Source: CAD feature listing. Evaluate the final solid. Frame: model axes, mm. Face numbers are marked on the shaded views. A direction names the side the tool comes from. Round coordinates to 2 decimals unless told otherwise and drop trailing zeros. Write each loop counter-clockwise with the first axis right and the second up, starting at its lowest first coordinate (ties: lowest second). Pieces come first, ordered by that corner, then holes.
```python
from build123d import *

# Parameters (mm, degrees)
SKETCH1_W           = 50
SKETCH1_H           = 170
BOSS_EXTRUDE1_DEPTH = 55
SKETCH2_W           = 34
SKETCH2_H           = 27
CUT_EXTRUDE1_DEPTH  = 181.416185527
SKETCH3_W           = 10
SKETCH3_H           = 24
SKETCH3_R           = 4.25
SKETCH3_R_2         = 1
CUT_EXTRUDE2_DEPTH  = 186.539753153
SKETCH4_W           = 2
SKETCH4_H           = 24
CUT_EXTRUDE3_DEPTH  = 178.623196683
SKETCH5_W           = 6.25
SKETCH5_H           = 11.25
CUT_EXTRUDE4_DEPTH  = 186.539753153
SKETCH6_W           = 38
SKETCH6_H           = 10
CUT_EXTRUDE5_DEPTH  = 181.416185527
SKETCH8_W           = 13.25
SKETCH8_H           = 2.25
CUT_EXTRUDE7_DEPTH  = 186.539753153
SKETCH9_W           = 34
SKETCH9_H           = 35.25
CUT_EXTRUDE8_DEPTH  = 179.297679458
SKETCH11_W          = 13.25
SKETCH11_H          = 20.25
CUT_EXTRUDE9_DEPTH  = 184.480414486
SKETCH12_W          = 28.5
SKETCH12_H          = 15
BOSS_EXTRUDE2_DEPTH = 8
SKETCH14_W          = 34
SKETCH14_H          = 15
SKETCH14_H_2        = 10.25
BOSS_EXTRUDE3_DEPTH = 13.25
SKETCH16_R          = 4.5
SKETCH16_R_2        = 2.5
CUT_EXTRUDE13_DEPTH = 8


with BuildPart() as part:
    # Sketch1 → Boss-Extrude1 (new body)
    with BuildSketch(Plane.XY):
        with Locations((0, -85)):
            Rectangle(SKETCH1_W, SKETCH1_H)
    extrude(amount=-BOSS_EXTRUDE1_DEPTH)

    # Sketch2 → Cut-Extrude1 (cut, through all)
    with BuildSketch(Plane.XY):
        with Locations((0, -13.5)):
            Rectangle(SKETCH2_W, SKETCH2_H)
    extrude(amount=-CUT_EXTRUDE1_DEPTH, mode=Mode.SUBTRACT)

    # Sketch3 → Cut-Extrude2 (cut, through all)
    with BuildSketch(Plane(origin=(25, 0, 0), x_dir=(0, 0, -1), z_dir=(1, 0, 0))):
        with Locations((50, -12)):
            Rectangle(SKETCH3_W, SKETCH3_H)
        with Locations((5, -12)):
            Rectangle(SKETCH3_W, SKETCH3_H)
        with Locations(Location((27.5, -12.75, 0), (0, 0, 90))):
            Circle(SKETCH3_R)
        with Locations(Location((35.5, -12.75, 0), (0, 0, 90))):
            Circle(SKETCH3_R_2)
        with Locations(Location((27.5, -4.75, 0), (0, 0, 90))):
            Circle(SKETCH3_R_2)
        with Locations(Location((27.5, -20.75, 0), (0, 0, 90))):
            Circle(SKETCH3_R_2)
        with Locations(Location((19.5, -12.75, 0), (0, 0, 90))):
            Circle(SKETCH3_R_2)
    extrude(amount=-CUT_EXTRUDE2_DEPTH, mode=Mode.SUBTRACT)

    # Sketch4 → Cut-Extrude3 (cut, through all)
    with BuildSketch(Plane.XY.offset(-10)):
        with Locations((-18, -12)):
            Rectangle(SKETCH4_W, SKETCH4_H)
        with Locations((18, -12)):
            Rectangle(SKETCH4_W, SKETCH4_H)
    extrude(amount=-CUT_EXTRUDE3_DEPTH, mode=Mode.SUBTRACT)

    # Sketch5 → Cut-Extrude4 (cut, through all)
    with BuildSketch(Plane(origin=(25, 0, 0), x_dir=(0, 0, -1), z_dir=(1, 0, 0))):
        with BuildLine():
            Line((45, 0), (10, 0))
            Line((10, 0), (10, -12.75))
            Line((10, -12.75), (16.25, -12.75))
            ThreePointArc((16.25, -12.75), (27.5, -1.5), (38.75, -12.75))
            Line((38.75, -12.75), (45, -12.75))
            Line((45, -12.75), (45, 0))
        make_face()
        with Locations((13.125, -18.375)):
            Rectangle(SKETCH5_W, SKETCH5_H)
        with Locations((41.875, -18.375)):
            Rectangle(SKETCH5_W, SKETCH5_H)
    extrude(amount=-CUT_EXTRUDE4_DEPTH, mode=Mode.SUBTRACT)

    # Sketch6 → Cut-Extrude5 (cut, through all)
    with BuildSketch(Plane.XY):
        with Locations((0, -29)):
            Rectangle(SKETCH6_W, SKETCH6_H)
    extrude(amount=-CUT_EXTRUDE5_DEPTH, mode=Mode.SUBTRACT)

    # Sketch8 → Cut-Extrude7 (cut, through all)
    with BuildSketch(Plane(origin=(25, 0, 0), x_dir=(0, 0, -1), z_dir=(1, 0, 0))):
        with BuildLine():
            Line((27.5, -157.5), (27.5, -132.5))
            Line((27.5, -132.5), (13.25, -132.5))
            Line((13.25, -132.5), (13.25, -167.75))
            Line((13.25, -167.75), (17.25, -167.75))
            ThreePointArc((17.25, -167.75), (20.252155493, -160.502155493), (27.5, -157.5))
        make_face()
        with BuildLine():
            Line((41.75, -167.75), (41.75, -132.5))
            Line((41.75, -132.5), (27.5, -132.5))
            Line((27.5, -132.5), (27.5, -157.5))
            ThreePointArc((27.5, -157.5), (34.747844507, -160.502155493), (37.75, -167.75))
            Line((37.75, -167.75), (41.75, -167.75))
        make_face()
        with Locations((48.375, -168.875)):
            Rectangle(SKETCH8_W, SKETCH8_H)
        with Locations((6.625, -168.875)):
            Rectangle(SKETCH8_W, SKETCH8_H)
        with BuildLine():
            Line((17.25, -167.75), (13.25, -167.75))
            Line((13.25, -167.75), (13.25, -170))
            Line((13.25, -170), (17.5, -170))
            ThreePointArc((17.5, -170), (17.31269172, -168.881923142), (17.25, -167.75))
        make_face()
        with BuildLine():
            Line((41.75, -170), (41.75, -167.75))
            Line((41.75, -167.75), (37.75, -167.75))
            ThreePointArc((37.75, -167.75), (37.68730828, -168.881923142), (37.5, -170))
            Line((37.5, -170), (41.75, -170))
        make_face()
        with BuildLine():
            Line((27.5, -167.75), (27.5, -157.5))
            ThreePointArc((27.5, -157.5), (20.252155493, -160.502155493), (17.25, -167.75))
            Line((17.25, -167.75), (27.5, -167.75))
        make_face()
        with BuildLine():
            ThreePointArc((37.75, -167.75), (34.747844507, -160.502155493), (27.5, -157.5))
            Line((27.5, -157.5), (27.5, -167.75))
            Line((27.5, -167.75), (37.75, -167.75))
        make_face()
        with BuildLine():
            Line((27.5, -170), (27.5, -167.75))
            Line((27.5, -167.75), (17.25, -167.75))
            ThreePointArc((17.25, -167.75), (17.31269172, -168.881923142), (17.5, -170))
            Line((17.5, -170), (27.5, -170))
        make_face()
        with BuildLine():
            ThreePointArc((37.5, -170), (37.68730828, -168.881923142), (37.75, -167.75))
            Line((37.75, -167.75), (27.5, -167.75))
            Line((27.5, -167.75), (27.5, -170))
            Line((27.5, -170), (37.5, -170))
        make_face()
    extrude(amount=-CUT_EXTRUDE7_DEPTH, mode=Mode.SUBTRACT)

    # Sketch9 → Cut-Extrude8 (cut, through all)
    with BuildSketch(Plane.XY):
        with Locations((0, -150.125)):
            Rectangle(SKETCH9_W, SKETCH9_H)
    extrude(amount=-CUT_EXTRUDE8_DEPTH, mode=Mode.SUBTRACT)

    # Sketch11 → Cut-Extrude9 (cut, through all)
    with BuildSketch(Plane(origin=(25, 0, 0), x_dir=(0, 0, -1), z_dir=(1, 0, 0))):
        with BuildLine():
            ThreePointArc((17.25, -167.75), (20.252155493, -160.502155493), (27.5, -157.5))
            Line((27.5, -157.5), (27.5, -147.5))
            Line((27.5, -147.5), (13.25, -147.5))
            Line((13.25, -147.5), (13.25, -167.75))
            Line((13.25, -167.75), (17.25, -167.75))
        make_face()
        with BuildLine():
            Line((27.5, -147.5), (27.5, -157.5))
            ThreePointArc((27.5, -157.5), (34.747844507, -160.502155493), (37.75, -167.75))
            Line((37.75, -167.75), (41.75, -167.75))
            Line((41.75, -167.75), (41.75, -147.5))
            Line((41.75, -147.5), (27.5, -147.5))
        make_face()
        with Locations((48.375, -157.625)):
            Rectangle(SKETCH11_W, SKETCH11_H)
        with Locations((6.625, -157.625)):
            Rectangle(SKETCH11_W, SKETCH11_H)
    extrude(amount=-CUT_EXTRUDE9_DEPTH, mode=Mode.SUBTRACT)

    # Sketch12 → Boss-Extrude2 (add)
    with BuildSketch(Plane(origin=(25, 0, 0), x_dir=(0, 0, -1), z_dir=(1, 0, 0))):
        with Locations((27.5, -140)):
            Rectangle(SKETCH12_W, SKETCH12_H)
    boss_extrude2 = extrude(amount=-BOSS_EXTRUDE2_DEPTH)

    # Mirror1: Boss-Extrude2 across plane
    add(boss_extrude2.mirror(Plane(origin=(0, 0, 0), x_dir=(0, 0, 1), z_dir=(1, 0, 0))))

    # Sketch14 → Boss-Extrude3 (add)
    with BuildSketch(Plane.XY):
        with Locations((0, -140)):
            Rectangle(SKETCH14_W, SKETCH14_H)
        with Locations((0, -152.625)):
            Rectangle(SKETCH14_W, SKETCH14_H_2)
    boss_extrude3 = extrude(amount=-BOSS_EXTRUDE3_DEPTH)

    # Mirror2: Boss-Extrude3 across plane
    add(boss_extrude3.mirror(Plane.XY.offset(-27.5)))

    # Sketch16 → Cut-Extrude13 (cut)
    # profile 1 of 3: a face of its own
    with BuildSketch(Plane(origin=(25, 0, 0), x_dir=(0, 0, -1), z_dir=(1, 0, 0))):
        with Locations(Location((16.5, -135.75, 0), (0, 0, 90))):
            Circle(SKETCH16_R)
        with Locations((16.5, -135.75)):
            Circle(SKETCH16_R_2, mode=Mode.SUBTRACT)
    # profile 2 of 3: a face of its own
    with BuildSketch(Plane(origin=(25, 0, 0), x_dir=(0, 0, -1), z_dir=(1, 0, 0))):
        with Locations((16.5, -135.75)):
            Circle(SKETCH16_R_2)
    # profile 3 of 3: a face of its own
    with BuildSketch(Plane(origin=(25, 0, 0), x_dir=(0, 0, -1), z_dir=(1, 0, 0))):
        with Locations(Location((38.5, -135.75, 0), (0, 0, 90))):
            Circle(SKETCH16_R)
    cut_extrude13 = extrude(amount=-CUT_EXTRUDE13_DEPTH, mode=Mode.SUBTRACT)

    # Mirror3: Cut-Extrude13 across plane
    add(cut_extrude13.mirror(Plane(origin=(0, 0, 0), x_dir=(0, 0, 1), z_dir=(1, 0, 0))), mode=Mode.SUBTRACT)


solid = part.part
```
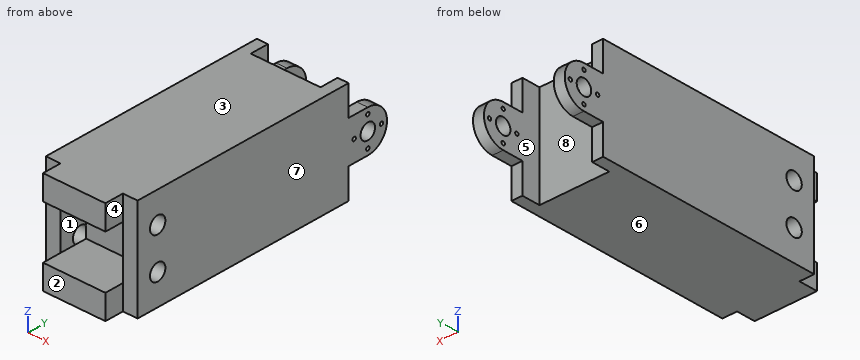
Q1. Set-up query: the marked faces 1, 2, 3, 4 and 5. Return all of +Z, -Z, +X, -X, +Y, -Y with unobstructed straight access to the full face (end or side cutting, diameter ignored); none if empty.
Q2. Pin query (flat end, axial travel): P1, Ø5, axis at x = -22.5, y = -20.5, coming from the -Z side; P2, Ø4, axis at x = -7.5, z = -44, coming from the +Y side; P3, Ø8, axis at y = -152.5, z = -50, coming from the -X side; P4, Ø1.4, axis at y = -135.5, z = -12.5, coming from the +X side. Return the tip coordinate at first contact, or that it passes through.
Q3. Section query C-C, the plane y = -144.5. Output: boundary loops of the cut face in (x, z).
Q4. Section query A-A, the plane z = -7.5. Output: boundary loops of the cut face in (x, y).
Q5. Line query: line 1 (Z direction, x = -20, y = -135); line 2 (Z direction, x = 10.5, y = -142); line 3 (Y direction, x = 21, z = -35). Output: solid intervals per line, ascending.
Q6. Section query B-B, the plane x = 10.5. Output: boundary loops of the cut face in (y, z), and give its area (3 significant figures).
Q7. Mould query, pull axis X, two halves, no side actions, for the marked faces 6, 7 and 8. Classes: pulls with the +X half, pulls with the -X half, needs draft (parallel to the pull), parting line crosses it, or undercut.
Filled in:
1. face 1: -Y
1. face 2: +Z, -Z, +X, -X, -Y
1. face 3: +Z, +X, -X, +Y, -Y
1. face 4: +Z, -Z, +X, -Y
1. face 5: +Z, -Z, +Y
2. P1: stops at z = -38.75
2. P2: stops at y = -34
2. P3: stops at x = -17
2. P4: stops at x = 25
3. outline: (-25, -55) - (25, -55) - (25, 0) - (-25, 0) - close; hole (-17, -41.75) - (17, -41.75) - (17, -13.25) - (-17, -13.25) - close
4. outline: (-25, -147.5) - (-17, -147.5) - (-17, -157.75) - (17, -157.75) - (17, -147.5) - (25, -147.5) - (25, -24) - (19, -24) - (19, -34) - (-19, -34) - (-19, -24) - (-25, -24) - close
5. line 1: z = -55 to -42.94, -34.06 to -20.94, -12.06 to 0
5. line 2: z = -55 to -41.75, -13.25 to 0
5. line 3: y = -147.5 to -138.58, -132.92 to -13.62, -11.88 to -4.36
6. outline: (-157.75, -55) - (-34, -55) - (-34, 0) - (-157.75, 0) - (-157.75, -13.25) - (-132.5, -13.25) - (-132.5, -41.75) - (-157.75, -41.75) - close
6. area: 6,090 mm2
7. face 6: needs draft
7. face 7: pulls with the +X half
7. face 8: undercut
